For this review, take the finished solid that the model builds, in its own axes (mm). Round coordinates to 2 decimals unless told otherwise and drop trailing zeros. Write each loop counter-clockwise with the first axis right and the second up, starting at its lowest first coordinate (ties: lowest second). Pieces come first, ordered by that corner, then holes. Notation, with made-up numbers: M 32.25,75.5 L 47.25,75.5 A6 ccw 47.25,83.5 Z; hole C 80.25,35 d2. An arc over 180 degrees is marked long. Answer in a Markdown table with one row per item.
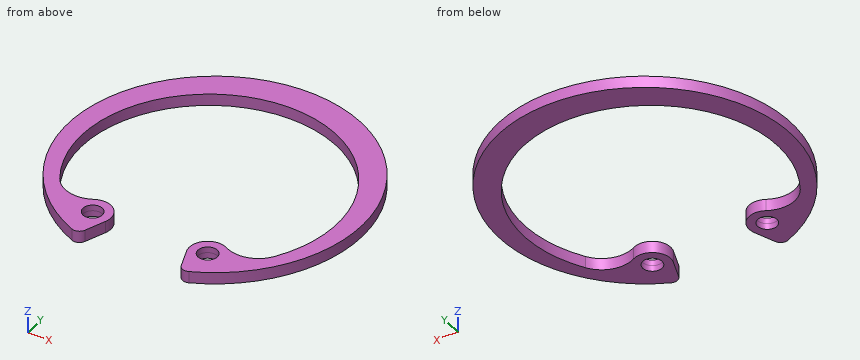
```python
from build123d import *

# Parameters (mm, degrees)
SKETCH3_R                = 1
BOSS_EXTRUDE1_DEPTH      = 0.6
BOSS_EXTRUDE1_DEPTH_BACK = 0.6
FILLET1_R                = 0.79375


with BuildPart() as part:
    # Sketch3 → Boss-Extrude1 (new body, two sides)
    with BuildSketch(Plane.XY) as boss_extrude1_sk:
        with BuildLine():
            Line((-4.20731071, -11.215994677), (-5.285853659, -14.091211839))
            ThreePointArc((-5.285853659, -14.091211839), (0, 15.05), (5.285853659, -14.091211839))
            Line((5.285853659, -14.091211839), (4.20731071, -11.215994677))
            ThreePointArc((4.20731071, -11.215994677), (4.738417429, -9.137470587), (6.87245355, -8.917865085))
            ThreePointArc((6.87245355, -8.917865085), (9.230393871, -9.214719738), (11.140467802, -7.800639534))
            ThreePointArc((11.140467802, -7.800639534), (0, 12.15), (-11.140467802, -7.800639534))
            ThreePointArc((-11.140467802, -7.800639534), (-9.230393871, -9.214719738), (-6.87245355, -8.917865085))
            ThreePointArc((-6.87245355, -8.917865085), (-4.738417429, -9.137470587), (-4.20731071, -11.215994677))
        make_face()
        with Locations((-5.962860358, -10.557458091)):
            Circle(SKETCH3_R, mode=Mode.SUBTRACT)
        with Locations((5.962860358, -10.557458091)):
            Circle(SKETCH3_R, mode=Mode.SUBTRACT)
    extrude(amount=BOSS_EXTRUDE1_DEPTH)
    extrude(boss_extrude1_sk.sketch, amount=-BOSS_EXTRUDE1_DEPTH_BACK)

    # Fillet1
    fillet1_edges = [part.edges().sort_by_distance(p)[0] for p in [
        (5.285853659, -14.091211839, 0),
        (-5.285853659, -14.091211839, 0),
    ]]
    fillet(fillet1_edges, radius=FILLET1_R)


solid = part.part
```
Q1. Take a section at B-B (z = 0.4). State how many separate pieces and enclosed holes the cut face has, then the cut area to 3 significant figures.
Found:
| item | result |
|---|---|
| separate pieces | 1 |
| enclosed holes | 2 |
| area | 186 mm² |
Q2. Take a section at C-C (x = 10). State the section outline as (y, z) points.
Found:
| item | result |
|---|---|
| outline | M -11.25,-0.6 L -8.9,-0.6 L -8.9,0.6 L -11.25,0.6 Z; M 7.5,-0.6 L 11.25,-0.6 L 11.25,0.6 L 7.5,0.6 Z |
Q3. Take a section at A-A (y = -2.25). State the section outline as (x, z) points, then the cut area to 3 significant figures.
Found:
| item | result |
|---|---|
| outline | M -14.88,-0.6 L -13.02,-0.6 L -13.02,0.6 L -14.88,0.6 Z; M 13.02,-0.6 L 14.88,-0.6 L 14.88,0.6 L 13.02,0.6 Z |
| area | 4.47 mm² |
Q4. Take a section at D-D (x = 0). State the section outline as (y, z) points, then the cut area to 3 significant figures.
Found:
| item | result |
|---|---|
| outline | M 12.15,-0.6 L 15.05,-0.6 L 15.05,0.6 L 12.15,0.6 Z |
| area | 3.48 mm² |
Q5. For probe 1 along Y at (x, z) = (-5.5, -0.1); probe 2 along X at (y, z) = (4, 0.2); probe 3 along X at (y, z) = (-12.25, -0.05), list the stretches that pass through material, from the lowest coordinate up.
Found:
| item | result |
|---|---|
| probe 1 | -13.8 to -11.44, -9.67 to -8.74, 10.94 to 14.01 |
| probe 2 | -14.51 to -12.12, 12.12 to 14.51 |
| probe 3 | -8.74 to -4.6, 4.6 to 8.74 |
